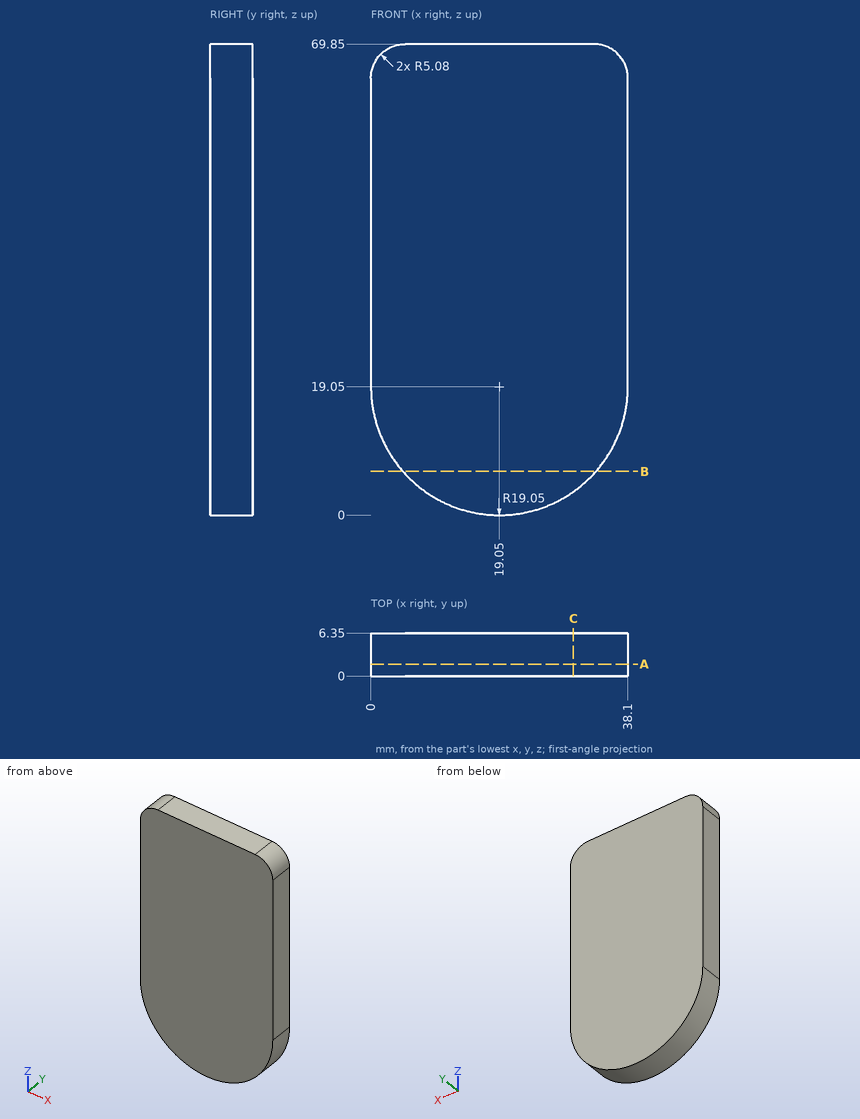
Drawing for the job (mm, zero at the part's lowest x, y, z). Round coordinates to 2 decimals unless told otherwise and drop trailing zeros. Order: outer loops, then holes, each group sorted by start corner. A loop starts at its lowest first (then second) coordinate and runs counter-clockwise, first axis right, second up. Notation, with made-up numbers: (31, -4) -> (86, -4) arc R26 cw to (86, 17) -> close; hole circle Ø1 at (-6.75, -21.75). An arc over 180 degrees is marked (long way). Write item = value, one per line. Start each with the question number.
(1) Pin check, flat tips, straight feed: P1, Ø1, axis at x = 16, y = 2.5, coming from the -Z side; P2, Ø1, axis at x = 27.5, y = 5, coming from the -Z side; P3, Ø2, axis at x = 30, y = 1.5, coming from the -Z side (3 decimals). Stop position of each tip, or through.
(2) Cut at C-C, the plane x = 30. List the corners of the cut face in (y, z).
(3) Cut at A-A, the plane y = 1.75. List the corners of the cut face in (x, z), then the cut area to 3 significant figures.
(4) Probe line 1 (Z direction, x = 19, y = 0.5); line 2 (Z direction, x = 32, y = 3.75); line 3 (X direction, y = 2.25, z = 15.5). List the from-to ranges inside material, lowest first. Write a range as [from, to].
(5) Cut at B-B, the plane z = 6.5. List the corners of the cut face in (x, y).
Model answer:
q1.P1 = 0.17
q1.P2 = 1.74
q1.P3 = 2.805
q2.outline = (0, 3.46) -> (6.35, 3.46) -> (6.35, 69.85) -> (0, 69.85) -> close
q3.outline = (0, 19.05) arc R19.05 ccw to (38.1, 19.05) -> (38.1, 64.77) arc R5.08 ccw to (33.02, 69.85) -> (5.08, 69.85) arc R5.08 ccw to (0, 64.77) -> close
q3.area = 2,490 mm2
q4.line_1 = [0, 69.85]
q4.line_2 = [5.08, 69.85]
q4.line_3 = [0.33, 37.77]
q5.outline = (4.72, 0) -> (33.38, 0) -> (33.38, 6.35) -> (4.72, 6.35) -> close
